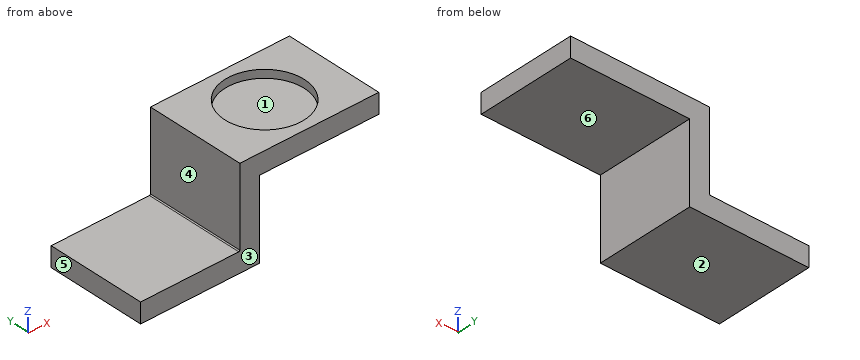
```python
from build123d import *

# Parameters (mm, degrees)
ESQUISSE1_W             = 30
ESQUISSE1_H             = 25
BOSS_EXTRU_2_DEPTH      = 5
ESQUISSE2_W             = 20
ESQUISSE2_H             = 25
BOSS_EXTRU_4_DEPTH      = 5
ESQUISSE3_W             = 5
ESQUISSE3_H             = 25
BOSS_EXTRU_5_DEPTH      = 30
CONG_1_R                = 0.25
ESQUISSE4_R             = 10
ENL_V_MAT_EXTRU_1_DEPTH = 2.03


with BuildPart() as part:
    # Esquisse1 → Boss.-Extru.2 (new body)
    with BuildSketch(Plane.XY):
        Rectangle(ESQUISSE1_W, ESQUISSE1_H)
    extrude(amount=BOSS_EXTRU_2_DEPTH)

    # Esquisse2 → Boss.-Extru.4 (add)
    with BuildSketch(Plane(origin=(15, 0, 0), x_dir=(0, 0, -1), z_dir=(1, 0, 0))):
        with Locations((-15, 0)):
            Rectangle(ESQUISSE2_W, ESQUISSE2_H)
    extrude(amount=-BOSS_EXTRU_4_DEPTH)

    # Esquisse3 → Boss.-Extru.5 (add)
    with BuildSketch(Plane(origin=(15, 0, 0), x_dir=(0, 0, -1), z_dir=(1, 0, 0))):
        with Locations((-22.5, 0)):
            Rectangle(ESQUISSE3_W, ESQUISSE3_H)
    extrude(amount=BOSS_EXTRU_5_DEPTH)

    # Congé1
    cong_1_edges = [part.edges().sort_by_distance(p)[0] for p in [
        (10, 0, 5),
    ]]
    fillet(cong_1_edges, radius=CONG_1_R)

    # Esquisse4 → Enlèv. mat.-Extru.1 (cut)
    with BuildSketch(Plane.XY.offset(25)):
        with Locations((27.5, 0)):
            Circle(ESQUISSE4_R)
    extrude(amount=-ENL_V_MAT_EXTRU_1_DEPTH, mode=Mode.SUBTRACT)


solid = part.part
```
Can you work these out from the model? Positions are in its coordinate system, mm. Face numbers are marked on the shaded views. A direction names the side the tool comes from. Round coordinates to 2 decimals unless told otherwise and drop trailing zeros. Loops run counter-clockwise (first coordinate to the right, second up) from the corner with the lowest first, then second, coordinate; pieces in that order, holes last.
Item 1: Suppose I cut it at D-D, the plane y = 0. Write out the boundary of the cut face in (x, z).
Item 2: If we mould it in two halves opening along Y, with no side actions, what happens to the marked faces 1, 2 and 3? For each: +Y half, -Y half, draft (parallel to the pull), parting line (faces both ways), or undercut.
Item 3: Suppose I cut it at A-A, the plane x = 33.5. Write out the boundary of the cut face in (y, z).
Item 4: Will these pins go through, and if not, where does the flat tip stop? pin 1 Ø6 at (y, z) = (4, 11.5) entering from -X; pin 2 Ø6 at (x, y) = (32, 0) entering from +Z; pin 3 Ø4 at (x, y) = (37, 3) entering from -Z.
Item 5: Which directions (+Z, -Z, +X, -X, +Y, -Y) give clear straight access to the entire face, cutting with the end or side of a thin tool? Please do the marked faces 4, 5 and 6.
Item 6: Please list where these lines run through material, in increasing order: L1, parallel to Y at x = 27.5, z = 23.7; L2, parallel to Z at x = 8.5, y = -9.25; L3, parallel to X at y = 6, z = 10.5.
Item 7: Suppose I cut it at B-B, the plane y = -10.75. Write out the boundary of the cut face in (x, z), then the cut area to 3 significant figures.
Item 8: Suppose I cut it at C-C, the plane z = 1.75. Write out the boundary of the cut face in (x, y).
Reported:
1. outline: (-15, 0) - (15, 0) - (15, 20) - (45, 20) - (45, 25) - (37.5, 25) - (37.5, 22.97) - (17.5, 22.97) - (17.5, 25) - (10, 25) - (10, 5.25) arc R0.25 cw to (9.75, 5) - (-15, 5) - close
2. face 1: undercut
2. face 2: draft
2. face 3: -Y half
3. outline: (-12.5, 20) - (12.5, 20) - (12.5, 25) - (8, 25) - (8, 22.97) - (-8, 22.97) - (-8, 25) - (-12.5, 25) - close
4. pin 1: stops at x = 10
4. pin 2: stops at z = 22.97
4. pin 3: stops at z = 20
5. face 4: +Z, -X, +Y, -Y
5. face 5: +Z, -Z, -X, +Y, -Y
5. face 6: -Z, +X, +Y, -Y
6. L1: y = -12.5 to -10, 10 to 12.5
6. L2: z = 0 to 5
6. L3: x = 10 to 15
7. outline: (-15, 0) - (15, 0) - (15, 20) - (45, 20) - (45, 25) - (10, 25) - (10, 5.25) arc R0.25 cw to (9.75, 5) - (-15, 5) - close
7. area: 400 mm2
8. outline: (-15, -12.5) - (15, -12.5) - (15, 12.5) - (-15, 12.5) - close
